```python
from build123d import *

# Parameters (mm, degrees)
SKETCH5_R           = 73.025
SKETCH5_R_2         = 3.175
PLATEBASE_DEPTH     = 6.35
PLATETOP_DEPTH      = 9.525
SKETCH9_R           = 73.025
SKETCH9_R_2         = 66.675
PLATEWALLS_DEPTH    = 9.525
SKETCH13_R          = 3.175
RIGHTTHRUHOLE_DEPTH = 6.35
SKETCH14_R          = 3.175
LEFTTHRUHOLE_DEPTH  = 6.35
BOSS_EXTRUDE1_DEPTH = 9.525
SKETCH16_R          = 4.765
INSERTHOLE_DEPTH    = 8.128
INSERTHOLES_COUNT   = 4


with BuildPart() as part:
    # Sketch5 → PlateBase (new body)
    with BuildSketch(Plane(origin=(0, 0, 0), x_dir=(1, 0, 0), z_dir=(0, 1, 0))):
        Circle(SKETCH5_R)
        with Locations((38.1, 38.1)):
            Circle(SKETCH5_R_2, mode=Mode.SUBTRACT)
        with Locations((38.1, -38.1)):
            Circle(SKETCH5_R_2, mode=Mode.SUBTRACT)
        with Locations((-38.1, 38.1)):
            Circle(SKETCH5_R_2, mode=Mode.SUBTRACT)
        with Locations((-38.1, -38.1)):
            Circle(SKETCH5_R_2, mode=Mode.SUBTRACT)
    extrude(amount=PLATEBASE_DEPTH)

    # Sketch6 → PlateTop (add)
    with BuildSketch(Plane(origin=(0, 6.35, 0), x_dir=(1, 0, 0), z_dir=(0, 1, 0))):
        with BuildLine():
            Line((-3.175, 0), (-3.175, 72.955945611))
            ThreePointArc((-3.175, 72.955945611), (-6.35605636, 72.747860261), (-9.525, 72.401139494))
            Line((-9.525, 72.401139494), (-9.525, 0))
            Line((-9.525, 0), (-9.525, -72.401139494))
            ThreePointArc((-9.525, -72.401139494), (-6.35605636, -72.747860261), (-3.175, -72.955945611))
            Line((-3.175, -72.955945611), (-3.175, 0))
        make_face()
        with BuildLine():
            Line((3.175, 72.955945611), (3.175, 0))
            Line((3.175, 0), (3.175, -72.955945611))
            ThreePointArc((3.175, -72.955945611), (6.35605636, -72.747860261), (9.525, -72.401139494))
            Line((9.525, -72.401139494), (9.525, 0))
            Line((9.525, 0), (9.525, 72.401139494))
            ThreePointArc((9.525, 72.401139494), (6.35605636, 72.747860261), (3.175, 72.955945611))
        make_face()
    extrude(amount=PLATETOP_DEPTH)

    # Sketch9 → PlateWalls (add)
    with BuildSketch(Plane(origin=(0, 6.35, 0), x_dir=(1, 0, 0), z_dir=(0, 1, 0))):
        Circle(SKETCH9_R)
        Circle(SKETCH9_R_2, mode=Mode.SUBTRACT)
    extrude(amount=PLATEWALLS_DEPTH)

    # Sketch13 → RightThruHole (cut)
    with BuildSketch(Plane(origin=(0, 6.35, 0), x_dir=(1, 0, 0), z_dir=(0, 1, 0))):
        with Locations((34.925, 0)):
            Circle(SKETCH13_R)
    extrude(amount=-RIGHTTHRUHOLE_DEPTH, mode=Mode.SUBTRACT)

    # Sketch14 → LeftThruHole (cut)
    with BuildSketch(Plane(origin=(0, 6.35, 0), x_dir=(1, 0, 0), z_dir=(0, 1, 0))):
        with Locations((-34.925, 0)):
            Circle(SKETCH14_R)
    extrude(amount=-LEFTTHRUHOLE_DEPTH, mode=Mode.SUBTRACT)

    # Sketch15 → Boss-Extrude1 (add)
    with BuildSketch(Plane(origin=(0, 6.35, 0), x_dir=(1, 0, 0), z_dir=(0, 1, 0))):
        with BuildLine():
            Line((-3.175, 63.5), (3.175, 63.5))
            Line((3.175, 63.5), (3.175, 66.599361859))
            ThreePointArc((3.175, 66.599361859), (0, 66.675), (-3.175, 66.599361859))
            Line((-3.175, 66.599361859), (-3.175, 63.5))
        make_face()
        with BuildLine():
            Line((-3.175, -63.5), (-3.175, -66.599361859))
            ThreePointArc((-3.175, -66.599361859), (0, -66.675), (3.175, -66.599361859))
            Line((3.175, -66.599361859), (3.175, -63.5))
            Line((3.175, -63.5), (-3.175, -63.5))
        make_face()
    extrude(amount=BOSS_EXTRUDE1_DEPTH)

    # Sketch16 → InsertHole (cut)
    with BuildSketch(Plane.XY.offset(73.025)):
        with Locations((0, 7.9375)):
            Circle(SKETCH16_R)
    inserthole = extrude(amount=-INSERTHOLE_DEPTH, mode=Mode.SUBTRACT)

    # InsertHoles: InsertHole ×4 about axis
    insertholes_axis = Axis((0, 0, 0), (0, 1, 0))
    for i in range(1, INSERTHOLES_COUNT):
        add(inserthole.rotate(insertholes_axis, i * 360 / INSERTHOLES_COUNT), mode=Mode.SUBTRACT)


solid = part.part
```
Work out the finished part from the listing and answer in its coordinate system (mm). A direction names the side the tool comes from. Give positions to 0.01 mm unless a question says otherwise; leave off trailing zeros. Write each loop counter-clockwise with the first axis right and the second up, starting at its lowest first coordinate (ties: lowest second). Pieces come first, ordered by that corner, then holes. Notation, with made-up numbers: (13, -35.75) -> (43, -35.75) arc R30 cw to (43, -6.75) -> close; hole circle Ø11 at (71, 78.25). An arc over 180 degrees is marked (long way). Write item = value, one per line.
Q1. Section D-D on z = 51.5 is taken. Determine the outline of the cut face in (x, y) (3 decimals), and give its area (3 significant figures).
Computed values:
outline = (-51.773, 0) -> (51.773, 0) -> (51.773, 15.875) -> (42.347, 15.875) -> (42.347, 6.35) -> (9.525, 6.35) -> (9.525, 15.875) -> (3.175, 15.875) -> (3.175, 6.35) -> (-3.175, 6.35) -> (-3.175, 15.875) -> (-9.525, 15.875) -> (-9.525, 6.35) -> (-42.347, 6.35) -> (-42.347, 15.875) -> (-51.773, 15.875) -> close
area = 958 mm^2
Q2. Consider line 1 along X through (y, z) = (3, 0) (3 decimals); line 2 along X through (y, z) = (4.5, 0); line 3 along X through (y, z) = (13.75, -35) (3 decimals). Determine where each line is inside the solid, lowest interval first.
Computed values:
line_1 = -73.025 to -38.1, -31.75 to 31.75, 38.1 to 73.025
line_2 = -64.9 to -38.1, -31.75 to 31.75, 38.1 to 64.9
line_3 = -64.091 to -56.75, -9.525 to -3.175, 3.175 to 9.525, 56.75 to 64.091
Q3. Section A-A on z = 0 is taken. State how many separate pieces and enclosed holes the cut face has, and give its area (3 significant figures).
Computed values:
separate_pieces = 5
enclosed_holes = 0
area = 956 mm^2
Q4. Flat-ended cylindrical pins translate along their axes: pin 1 Ø2 at (x, z) = (-19.5, 22) entering from +Y; pin 2 Ø1 at (y, z) = (5, 0.5) entering from -X; pin 3 Ø5 at (x, y) = (54.5, 8) entering from -Z; pin 4 Ø5.5 at (x, z) = (-34.925, 0) entering from -Y. Find the tip coordinate at first contact, or state that the pin passes through.
Computed values:
pin_1 = 6.35
pin_2 = -64.9
pin_3 = -51.27
pin_4 = through
Q5. For a pull along Z with two mould halves and no side action, classify faces 6 (the flat face through (-1, 0, -1)), 7 (the cylindrical face through (69.02, 3.71, -2.2)), 8 (the flat face through (0, 8, 64.897)) as pulls with the +Z half, pulls with the -Z half, needs draft (parallel to the pull), parting line crosses it, or undercut.
Computed values:
face_6 = needs draft
face_7 = undercut
face_8 = pulls with the +Z half
Q6. A tool of negligible diameter and unlimited length cuts with its end or side. For faces 1 (the cylindrical face through (-66.66, 13.16, -1.33)), 2 (the cylindrical face through (-69.02, 3.71, 2.2)), 3 (the flat face through (64.897, 5, 0)), 4 (the flat face through (-64.897, 5, 0)), 5 (the cylindrical face through (0.62, 12.66, -69.02)), from which of +Z, -Z, +X, -X, +Y, -Y can it reach the whole face along a straight path? Write none if from no direction.
Computed values:
face_1 = +Y
face_2 = -X
face_3 = +X, +Y
face_4 = -X, +Y
face_5 = -Z
Q7. Section C-C on z = -38.1 is taken. Determine the outline of the cut face in (x, y) (3 decimals).
Computed values:
outline = (-62.298, 0) -> (-41.275, 0) -> (-41.275, 6.35) -> (-54.717, 6.35) -> (-54.717, 15.875) -> (-62.298, 15.875) -> close; (-34.925, 0) -> (34.925, 0) -> (34.925, 6.35) -> (9.525, 6.35) -> (9.525, 15.875) -> (3.175, 15.875) -> (3.175, 6.35) -> (-3.175, 6.35) -> (-3.175, 15.875) -> (-9.525, 15.875) -> (-9.525, 6.35) -> (-34.925, 6.35) -> close; (41.275, 0) -> (62.298, 0) -> (62.298, 15.875) -> (54.717, 15.875) -> (54.717, 6.35) -> (41.275, 6.35) -> close
